Input: part model. Units: mm. Frame: model coordinates. A direction names the side the tool comes from. Give positions to 0.01 mm unless a question says otherwise; leave off trailing zeros. Loops run counter-clockwise (first coordinate to the right, second up) from the corner with the lowest first, then second, coordinate; pieces in that order, holes last.
from build123d import *

# Parameters (mm, degrees)
SKETCH_1_R      = 1.6
EXTRUDE_1_DEPTH = 8.5
SKETCH_2_R      = 2.6
EXTRUDE_2_DEPTH = 1
FILLET_1_R      = 1


with BuildPart() as part:
    # Эскиз1 → Бобышка-Вытянуть1 (new body)
    with BuildSketch(Plane.XY):
        Circle(SKETCH_1_R)
    extrude(amount=EXTRUDE_1_DEPTH)

    # Эскиз2 → Бобышка-Вытянуть2 (add)
    with BuildSketch(Plane.XY):
        Circle(SKETCH_2_R)
    extrude(amount=EXTRUDE_2_DEPTH)

    # Скругление1
    fillet_1_edges = [part.edges().sort_by_distance(p)[0] for p in [
        (-1.6, 0, 1),
    ]]
    fillet(fillet_1_edges, radius=FILLET_1_R - 0.0001)  # a hair under: the kernel refuses the full size


solid = part.part
(1) Reachability of faces 1 (the flat face through (0, 0, 0)), 2 (the cylindrical face through (-1.27, -0.97, 5.2)) from +Z, -Z, +X, -X, +Y, -Y: full face, straight path, thin tool, end or side. Return the list, or none.
Values follow:
face 1: -Z, +X, -X, +Y, -Y
face 2: +Z
(2) Cut plane C-C (z = 3.5). Return the cut outline in (x, y), and give its area (3 significant figures).
Values follow:
outline: circle Ø3.2 at (0, 0)
area: 8.04 mm2
(3) Pin query (flat end, axial travel): pin 1 Ø1 at (y, z) = (-1, 4) entering from -X; pin 2 Ø1 at (x, z) = (0.5, 6) entering from -Y; pin 3 Ø1.5 at (y, z) = (1, 4) entering from +X. Return the tip coordinate at first contact, or that it passes through.
Values follow:
pin 1: stops at x = -1.52
pin 2: stops at y = -1.6
pin 3: stops at x = 1.58
(4) Ray query, probe 1 along Z at (x, y) = (1.4, 1); probe 2 along X at (y, z) = (0.85, 1.75); probe 3 along Z at (x, y) = (-1.25, -1.65). Return the intervals inside material, ascending.
Values follow:
probe 1: z = 0 to 1.52
probe 2: x = -1.39 to 1.39
probe 3: z = 0 to 1.15
